The listing builds one solid part. Answer for the finished solid, in the listing's coordinates (mm). A direction names the side the tool comes from. Coordinates: 2 decimals unless noted, no trailing zeros. Write each loop counter-clockwise with the first axis right and the second up, starting at its lowest first coordinate (ties: lowest second). Pieces come first, ordered by that corner, then holes.
from build123d import *

# Parameters (mm, degrees)
SKETCH1_W           = 15
SKETCH1_H           = 35
BOSS_EXTRUDE1_DEPTH = 1.5
SKETCH2_W           = 9
SKETCH2_H           = 5
BOSS_EXTRUDE2_DEPTH = 4
FILLET1_R           = 0.2
SKETCH3_R           = 1.25
BOSS_EXTRUDE3_DEPTH = 2
FILLET2_R           = 1
SKETCH4_W           = 3
SKETCH4_H           = 3
BOSS_EXTRUDE4_DEPTH = 1
SKETCH5_R           = 2.5
BOSS_EXTRUDE5_DEPTH = 7.5
SKETCH6_W           = 2.4
SKETCH6_H           = 2.4
BOSS_EXTRUDE6_DEPTH = 2
FILLET3_R           = 0.1
SKETCH7_R           = 0.375
BOSS_EXTRUDE7_DEPTH = 5
FILLET4_R           = 0.2
SKETCH8_R           = 1.5
CUT_EXTRUDE1_DEPTH  = 21.46338193


with BuildPart() as part:
    # Sketch1 → Boss-Extrude1 (new body)
    with BuildSketch(Plane(origin=(0, 0, 0), x_dir=(1, 0, 0), z_dir=(0, 1, 0))):
        Rectangle(SKETCH1_W, SKETCH1_H)
    extrude(amount=BOSS_EXTRUDE1_DEPTH)

    # Sketch2 → Boss-Extrude2 (add)
    with BuildSketch(Plane(origin=(0, 1.5, 0), x_dir=(1, 0, 0), z_dir=(0, 1, 0))):
        with Locations((0, -15)):
            Rectangle(SKETCH2_W, SKETCH2_H)
    extrude(amount=BOSS_EXTRUDE2_DEPTH)

    # Fillet1
    fillet1_edges = [part.edges().sort_by_distance(p)[0] for p in [
        (4.5, 3.5, 17.5),
        (4.5, 3.5, 12.5),
        (-4.5, 3.5, 17.5),
        (-4.5, 3.5, 12.5),
    ]]
    fillet(fillet1_edges, radius=FILLET1_R)

    # Sketch3 → Boss-Extrude3 (add)
    with BuildSketch(Plane(origin=(0, 5.5, 0), x_dir=(1, 0, 0), z_dir=(0, 1, 0))):
        with Locations(Location((-1.9, -15, 0), (0, 0, 270))):
            Circle(SKETCH3_R)
        with Locations(Location((1.9, -15, 0), (0, 0, 90))):
            Circle(SKETCH3_R)
    extrude(amount=BOSS_EXTRUDE3_DEPTH)

    # Fillet2
    fillet2_edges = [part.edges().sort_by_distance(p)[0] for p in [
        (-1.9, 7.5, 13.75),
        (1.9, 7.5, 16.25),
    ]]
    fillet(fillet2_edges, radius=FILLET2_R)

    # Sketch4 → Boss-Extrude4 (add)
    with BuildSketch(Plane.XZ):
        with Locations((-5, 11)):
            Rectangle(SKETCH4_W, SKETCH4_H)
    extrude(amount=BOSS_EXTRUDE4_DEPTH)

    # Sketch5 → Boss-Extrude5 (add)
    with BuildSketch(Plane.XZ):
        with Locations(Location((2.5, 10.5, 0), (0, 0, 90))):
            Circle(SKETCH5_R)
    extrude(amount=BOSS_EXTRUDE5_DEPTH)

    # Sketch6 → Boss-Extrude6 (add)
    with BuildSketch(Plane.XZ):
        with Locations((-3.8, -14.3)):
            Rectangle(SKETCH6_W, SKETCH6_H)
        with Locations((-1.3, -14.3)):
            Rectangle(SKETCH6_W, SKETCH6_H)
        with Locations((1.2, -14.3)):
            Rectangle(SKETCH6_W, SKETCH6_H)
        with Locations((3.7, -14.3)):
            Rectangle(SKETCH6_W, SKETCH6_H)
    extrude(amount=BOSS_EXTRUDE6_DEPTH)

    # Fillet3
    fillet3_edges = [part.edges().sort_by_distance(p)[0] for p in [
        (-2.5, -1, -15.5),
        (-0.1, -1, -15.5),
        (-0.1, -1, -13.1),
        (-2.5, -1, -13.1),
        (0, -1, -15.5),
        (2.4, -1, -15.5),
        (2.4, -1, -13.1),
        (0, -1, -13.1),
        (2.5, -1, -15.5),
        (4.9, -1, -15.5),
        (4.9, -1, -13.1),
        (2.5, -1, -13.1),
        (-2.6, -1, -15.5),
        (-2.6, -1, -13.1),
        (-5, -1, -13.1),
        (-5, -1, -15.5),
    ]]
    fillet(fillet3_edges, radius=FILLET3_R)

    # Sketch7 → Boss-Extrude7 (add)
    with BuildSketch(Plane.XZ.offset(2)):
        with Locations(Location((-3.8, -14.3, 0), (0, 0, 270))):
            Circle(SKETCH7_R)
        with Locations(Location((-1.3, -14.3, 0), (0, 0, 90))):
            Circle(SKETCH7_R)
        with Locations(Location((1.2, -14.3, 0), (0, 0, 90))):
            Circle(SKETCH7_R)
        with Locations(Location((3.7, -14.3, 0), (0, 0, 90))):
            Circle(SKETCH7_R)
    extrude(amount=BOSS_EXTRUDE7_DEPTH)

    # Fillet4
    fillet4_edges = [part.edges().sort_by_distance(p)[0] for p in [
        (-3.8, -7, -13.925),
        (-1.3, -7, -14.675),
        (1.2, -7, -14.675),
        (3.7, -7, -14.675),
    ]]
    fillet(fillet4_edges, radius=FILLET4_R)

    # Sketch8 → Cut-Extrude1 (cut, through all)
    with BuildSketch(Plane.XZ):
        with Locations(Location((0, -8.5, 0), (0, 0, 270))):
            Circle(SKETCH8_R)
    extrude(amount=-CUT_EXTRUDE1_DEPTH, mode=Mode.SUBTRACT)


solid = part.part
1. Flat-ended cylindrical pins translate along their axes: P1, Ø3, axis at x = 4, z = 2.5, coming from the -Y side; P2, Ø1, axis at y = -1, z = -14.5, coming from the -X side; P3, Ø7.5, axis at x = 0.5, z = -5.5, coming from the +Y side. Find the tip coordinate at first contact, or state that the pin passes through.
Results found:
P1: stops at y = 0
P2: stops at x = -5
P3: stops at y = 1.5
2. Find the intervals of material crossed by L1, parallel to X at y = 0.55, z = -8.5; L2, parallel to Y at x = 6.5, z = 4; L3, parallel to X at y = 0.5, z = -8, in increasing order.
Results found:
L1: x = -7.5 to -1.5, 1.5 to 7.5
L2: y = 0 to 1.5
L3: x = -7.5 to -1.41, 1.41 to 7.5
3. A tool of negligible diameter and unlimited length cuts with its end or side. For faces 5 (the flat face through (-3.5, -0.5, 11)), 6 (the flat face through (3, -2, -14)), 7 (the flat face through (0, 5.5, 15)), 8 (the flat face through (-6.5, -0.5, 11)), 9 (the flat face through (-4.5, 3, 15)), from which of +Z, -Z, +X, -X, +Y, -Y can it reach the whole face along a straight path? Write none if from no direction.
Results found:
face 5: +Z, -Y
face 6: -Y
face 7: +Y
face 8: +Z, -Z, -X, -Y
face 9: +Z, -Z, -X, +Y
4. Section A-A on z = -8.5 is taken. Give the vertices of the cut face in (x, y), then the cut area to 3 significant figures.
Results found:
outline: (-7.5, 0) - (-1.5, 0) - (-1.5, 1.5) - (-7.5, 1.5) - close; (1.5, 0) - (7.5, 0) - (7.5, 1.5) - (1.5, 1.5) - close
area: 18.0 mm2
5. Section B-B on y = 2.5 is taken. Give the vertices of the cut face in (x, z).
Results found:
outline: (-4.5, 12.7) arc R0.2 ccw to (-4.3, 12.5) - (4.3, 12.5) arc R0.2 ccw to (4.5, 12.7) - (4.5, 17.3) arc R0.2 ccw to (4.3, 17.5) - (-4.3, 17.5) arc R0.2 ccw to (-4.5, 17.3) - close
6. Section D-D on z = 10.5 is taken. Give the vertices of the cut face in (x, y).
Results found:
outline: (-7.5, 0) - (-6.5, 0) - (-6.5, -1) - (-3.5, -1) - (-3.5, 0) - (0, 0) - (0, -7.5) - (5, -7.5) - (5, 0) - (7.5, 0) - (7.5, 1.5) - (-7.5, 1.5) - close
7. For a pull along Z with two mould halves and no side action, classify faces 1 (the flat face through (4.5, 3, 15)), 2 (the flat face through (0, 0, 0)), 3 (the flat face through (-1, -1, -13.1)), 4 (the flat face through (0, 3, 12.5)) as pulls with the +Z half, pulls with the -Z half, needs draft (parallel to the pull), parting line crosses it, or undercut.
Results found:
face 1: needs draft
face 2: undercut
face 3: pulls with the +Z half
face 4: pulls with the -Z half
8. Section C-C on y = -5.75 is taken. Give the vertices of the cut face in (x, z) (3 decimals).
Results found:
outline: circle Ø0.75 at (-3.8, -14.3); circle Ø0.75 at (-1.3, -14.3); circle Ø5 at (2.5, 10.5); circle Ø0.75 at (1.2, -14.3); circle Ø0.75 at (3.7, -14.3)
